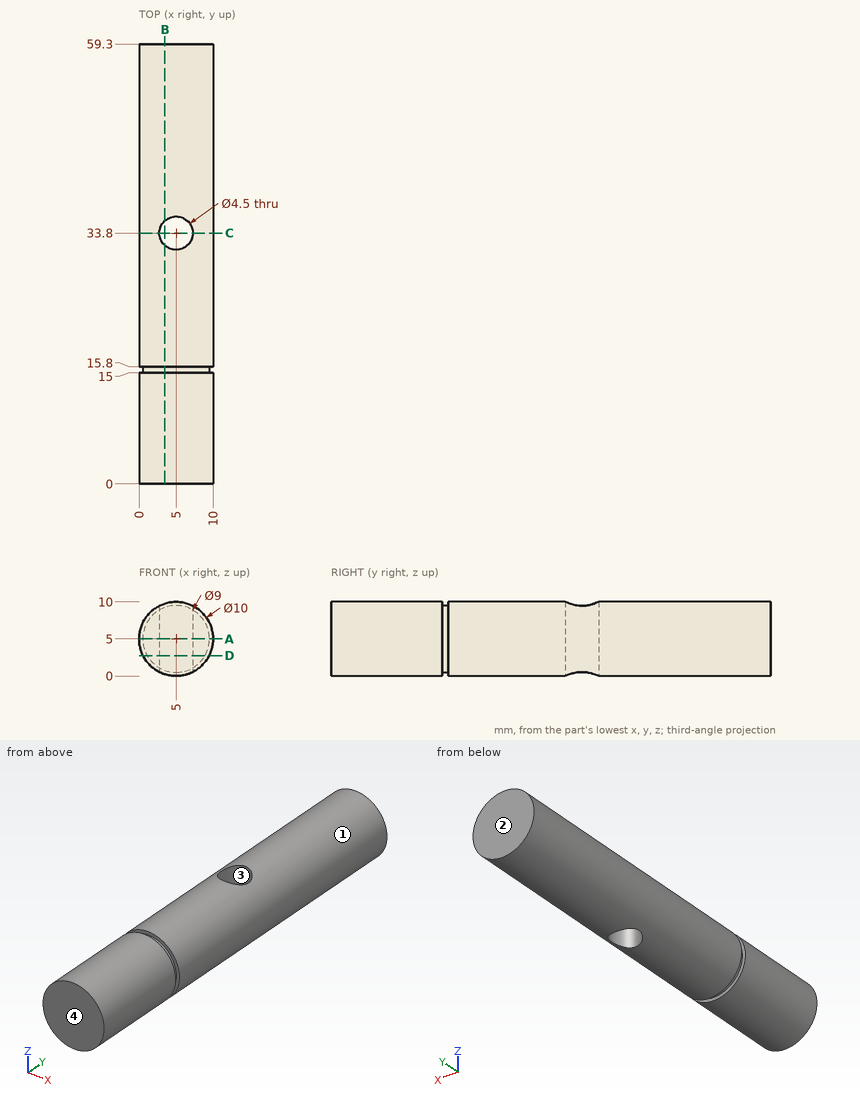
Answer from the drawing. Dimensions are ordinates in mm from the lowest x, y and z of the part. Round coordinates to 2 decimals unless told otherwise and drop trailing zeros. Order: outer loops, then holes, each group sorted by start corner. A loop starts at its lowest first (then second) coordinate and runs counter-clockwise, first axis right, second up.
1) The part is cut by section B-B on x = 3.5. Write down the section's boundary in (y, z).
2) Straight lines are drawn through the part: L1, parallel to Y at x = 5, z = 7.75; L2, parallel to Y at x = 0.5, z = 7; L3, parallel to X at y = 33.8, z = 6.25. For each, find the intervals that lie inside material, in ascending order.
3) Flat-ended cylindrical pins translate along their axes: pin 1 (2 mm diameter, centred on x = 8.5, y = 34, fed in from +Z); pin 2 (1.5 mm diameter, centred on y = 39.5, z = 8.5, fed in from +X); pin 3 (2 mm diameter, centred on y = 28.5, z = 3.5, fed in from +X). Find the tip coordinate at first contact, or state that the pin passes through.
4) The part is cut by section D-D on z = 2.75. Write down the section's boundary in (x, y).
5) The part is cut by section C-C on y = 33.8. Write down the section's boundary in (x, z).
6) The mould has two halves that part along Y. Classify the marked faces 1, 2, 3 and 4: released by +Y, released by -Y, zero draft, split by the parting line, or undercut.
7) The part is cut by section A-A on z = 5. Write down the section's boundary in (x, y).
Resolved:
1. outline: (0, 0.23) - (15, 0.23) - (15, 0.76) - (15.8, 0.76) - (15.8, 0.23) - (32.12, 0.23) - (32.12, 9.77) - (15.8, 9.77) - (15.8, 9.24) - (15, 9.24) - (15, 9.77) - (0, 9.77) - close; (35.48, 0.23) - (59.3, 0.23) - (59.3, 9.77) - (35.48, 9.77) - close
2. L1: y = 0 to 31.55, 36.05 to 59.3
2. L2: y = 0 to 15, 15.8 to 59.3
2. L3: x = 0.16 to 2.75, 7.25 to 9.84
3. pin 1: stops at z = 9.33
3. pin 2: stops at x = 9.18
3. pin 3: stops at x = 9.97
4. outline: (0.53, 0) - (9.47, 0) - (9.47, 15) - (8.9, 15) - (8.9, 15.8) - (9.47, 15.8) - (9.47, 59.3) - (0.53, 59.3) - (0.53, 15.8) - (1.1, 15.8) - (1.1, 15) - (0.53, 15) - close; hole circle Ø4.5 at (5, 33.8)
5. outline: (2.75, 0.53) - (2.75, 9.47) arc R5 ccw to start; (7.25, 0.53) arc R5 ccw to (7.25, 9.47) - close
6. face 1: zero draft
6. face 2: released by +Y
6. face 3: undercut
6. face 4: released by -Y
7. outline: (0, 0) - (10, 0) - (10, 15) - (9.5, 15) - (9.5, 15.8) - (10, 15.8) - (10, 59.3) - (0, 59.3) - (0, 15.8) - (0.5, 15.8) - (0.5, 15) - (0, 15) - close; hole circle Ø4.5 at (5, 33.8)
